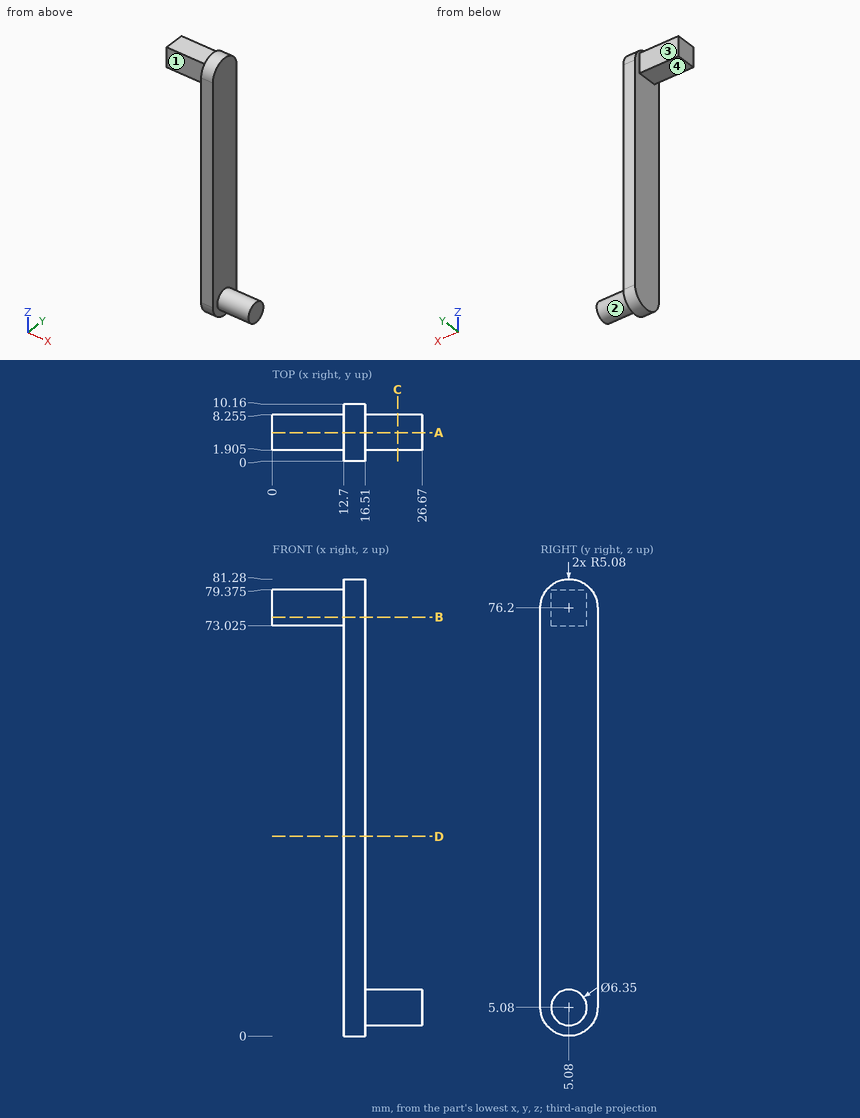
Can you work these out from the drawing? Everything is in mm from the part's minimum corner. A direction names the side the tool comes from. Coordinates: 2 decimals unless noted, no trailing zeros. Loops run counter-clockwise (first coordinate to the right, second up) from the corner with the lowest first, then second, coordinate; pieces in that order, holes last.
1) Imagine slicing it at D-D (z = 35.5). List the corners of the cut face in (x, y) for me.
Reported:
outline: (12.7, 0) - (16.51, 0) - (16.51, 10.16) - (12.7, 10.16) - close
2) Which directions (+Z, -Z, +X, -X, +Y, -Y) give clear straight access to the entire face, cutting with the end or side of a thin tool? Please do the marked faces 1, 2, 3 and 4.
Reported:
face 1: +Z, -Z, -X, -Y
face 2: +X
face 3: +Z, -Z, -X, +Y
face 4: -Z, -X, +Y, -Y
3) Imagine slicing it at B-B (z = 74.5). List the corners of the cut face in (x, y) for me (3 decimals).
Reported:
outline: (0, 1.905) - (12.7, 1.905) - (12.7, 0) - (16.51, 0) - (16.51, 10.16) - (12.7, 10.16) - (12.7, 8.255) - (0, 8.255) - close
4) Imagine slicing it at C-C (x = 22.25). List the corners of the cut face in (y, z) for me (3 decimals).
Reported:
outline: circle Ø6.35 at (5.08, 5.08)
5) Please list where these lines run through material, in increasing order: line 1 along Z through (x, y) = (1, 4) (3 decimals); line 2 along X through (y, z) = (5.25, 53); line 3 along X through (y, z) = (5.25, 4).
Reported:
line 1: z = 73.025 to 79.375
line 2: x = 12.7 to 16.51
line 3: x = 12.7 to 26.67
6) Will these pins go through, and if not, where does the flat tip stop? pin 1 Ø5 at (x, z) = (9, 77.5) entering from -Y (3 decimals); pin 2 Ø5 at (x, y) = (4, 4) entering from +Z (3 decimals); pin 3 Ø3 at (x, y) = (23.5, 3) entering from -Z.
Reported:
pin 1: stops at y = 1.905
pin 2: stops at z = 79.375
pin 3: stops at z = 1.96
7) Imagine slicing it at A-A (y = 5.08). List the corners of the cut face in (x, z) for me (3 decimals).
Reported:
outline: (0, 73.025) - (12.7, 73.025) - (12.7, 0) - (16.51, 0) - (16.51, 1.905) - (26.67, 1.905) - (26.67, 8.255) - (16.51, 8.255) - (16.51, 81.28) - (12.7, 81.28) - (12.7, 79.375) - (0, 79.375) - close
